Autodesk Inventor part; units mm, degrees
ref_plane "YZ Plane" through (0, 0, 0) normal (1, 0, 0) x (0, 1, 0)
ref_plane "XZ Plane" through (0, 0, 0) normal (0, 1, 0) x (-1, 0, 0)
ref_plane "XY Plane" through (0, 0, 0) normal (0, 0, 1) x (1, 0, 0)
sketch "Sketch1" plane through (0, 0, 0) normal (0, 0, 1) x (1, 0, 0)
  line L0 (0, 0) -> (0, 3)
  arc A0 (32.339, 0) -> (7.661, 0) centre (20, -2) ccw
  line L1 (0, 0) -> (7.661, 0)
  arc A1 (34.2916, 4) -> (5.3286, 3) centre (20, -2) ccw
  line L2 (0, 3) -> (5.3286, 3)
  line L3 (40, 0) -> (40, 3)
  line L4 (32.339, 0) -> (40, 0)
  line L5 (20, -2) -> (20, 11.991)
  line L6 (40, 0) -> (40, 3)
  line L7 (40, 0) -> (32.339, 0)
  arc A2 (34.6714, 3) -> (5.7084, 4) centre (20, -2) ccw
  line L8 (40, 3) -> (34.6714, 3)
  dimension "d12" = 20
  dimension "d14" = 25
  dimension "d38" = 2
  dimension "d40" = 3
  dimension "d41" = 40
  dimension "d57" = 3
extrude "Extrusion1" add sketch "Sketch1" along normal blind 40
sketch "Sketch3" plane through (0, 3, 0) normal (0, 1, 0) x (1, 0, 0)
  line L0 (5.3286, 0) -> (0, 0)
  line L1 (5.3286, -40) -> (0, -40)
  line L2 (0, 0) -> (0, -40)
  line L3 (40, 0) -> (40, -40)
  point P0 (3, -10)
  point P1 (3, -30)
  point P2 (37, -10)
  point P3 (37, -30)
  dimension "d42" = 10
  dimension "d43" = 20
  dimension "d45" = 20
  dimension "d53" = 3
  dimension "d54" = 3
  dimension "d55" = 3
  dimension "d56" = 3
hole "Hole2" at (3, 3, 10) at (3, 3, 30) at (37, 3, 10) at (37, 3, 30) direction (0, -1, 0) diameter 2.459 end through all
Source: CAD feature listing. Evaluate the final solid. Frame: model axes, mm. A direction names the side the tool comes from. Give positions to 0.01 mm unless a question says otherwise; leave off trailing zeros. Order: outer loops, then holes, each group sorted by start corner. A loop starts at its lowest first (then second) coordinate and runs counter-clockwise, first axis right, second up. Notation, with made-up numbers: (-7.75, -35.5) -> (27.25, -35.5) arc R27 ccw to (27.25, -11.5) -> close; hole circle Ø11 at (24, 31). An arc over 180 degrees is marked (long way). Use a Markdown table: item, result.
1) Reachability of faces 4 (the flat face through (3, 3, 20)), 5 (the cylindrical face through (35.78, 1.48, 9.84)) from +Z, -Z, +X, -X, +Y, -Y: full face, straight path, thin tool, end or side. Return the list, or none.
Answer list:
| item | result |
|---|---|
| face 4 | +Z, -Z, -X, +Y |
| face 5 | +Y, -Y |
2) Contact query for flat-ended pins moving along their axis: P1, Ø6, axis at x = 13, z = 25.5, coming from the -Y side; P2, Ø4.5, axis at x = 38, z = 28, coming from the +Y side; P3, Ø1.5, axis at y = 9.5, z = 15, coming from the -X side. Output: stop coordinate, or through.
Answer list:
| item | result |
|---|---|
| P1 | y = 5.5 |
| P2 | y = 3 |
| P3 | x = 8.83 |
3) Section query A-A, the plane z = 10. Return the cut outline in (x, y).
Answer list:
| item | result |
|---|---|
| outline | (0, 0) -> (1.77, 0) -> (1.77, 3) -> (0, 3) -> close; (4.23, 0) -> (7.66, 0) arc R12.5 cw to (32.34, 0) -> (35.77, 0) -> (35.77, 3) -> (34.67, 3) arc R15.5 ccw to (34.29, 4) arc R15.5 ccw to (5.33, 3) -> (4.23, 3) -> close; (38.23, 0) -> (40, 0) -> (40, 3) -> (38.23, 3) -> close |
4) Section query C-C, the plane y = 9. Return the cut outline in (x, z).
Answer list:
| item | result |
|---|---|
| outline | (9.08, 0) -> (14.06, 0) -> (14.06, 40) -> (9.08, 40) -> close; (25.94, 0) -> (30.92, 0) -> (30.92, 40) -> (25.94, 40) -> close |
5) Section query B-B, the plane x = 3. Return the cut outline in (y, z).
Answer list:
| item | result |
|---|---|
| outline | (0, 0) -> (3, 0) -> (3, 8.77) -> (0, 8.77) -> close; (0, 11.23) -> (3, 11.23) -> (3, 28.77) -> (0, 28.77) -> close; (0, 31.23) -> (3, 31.23) -> (3, 40) -> (0, 40) -> close |
6) Mould query, pull axis X, two halves, no side actions, for faces 1 (the flat face through (0, 1, 20)), 2 (the cylindrical face through (19.8, 10.5, 19.7)), 3 (the flat face through (37, 3, 20)). Classes: +X half, -X half, draft (parallel to the pull), parting line (faces both ways), or undercut.
Answer list:
| item | result |
|---|---|
| face 1 | -X half |
| face 2 | undercut |
| face 3 | draft |
7) Ray query, line 1 along Z through (x, y) = (3, 1.7); line 2 along X through (y, z) = (1.55, 30); line 3 along X through (y, z) = (1.7, 30). Return the intervals inside material, ascending. Write a range as [from, to].
Answer list:
| item | result |
|---|---|
| line 1 | [0, 8.77], [11.23, 28.77], [31.23, 40] |
| line 2 | [0, 1.77], [4.23, 8.01], [31.99, 35.77], [38.23, 40] |
| line 3 | [0, 1.77], [4.23, 8.06], [31.94, 35.77], [38.23, 40] |
8) Section query D-D, the plane z = 19.5. Return the cut outline in (x, y), then the cut area to 3 significant figures.
Answer list:
| item | result |
|---|---|
| outline | (0, 0) -> (7.66, 0) arc R12.5 cw to (32.34, 0) -> (40, 0) -> (40, 3) -> (34.67, 3) arc R15.5 ccw to (34.29, 4) arc R15.5 ccw to (5.33, 3) -> (0, 3) -> close |
| area | 149 mm² |
